Read the model definition and answer for the solid it produces. Units are mm, in the model's axes. Face numbers are marked on the shaded views. Coordinates: 2 decimals unless noted, no trailing zeros. Write each loop counter-clockwise with the first axis right and the second up, starting at its lowest first coordinate (ties: lowest second). Pieces come first, ordered by that corner, then holes.
(1) Section B-B on y = 0 is taken. Write down the section's boundary in (x, z).
(2) Section D-D on z = -10.5 is taken. Write down the section's boundary in (x, y).
(3) Section A-A on x = 10 is taken. Write down the section's boundary in (y, z), then the cut area to 3 significant figures.
(4) Find the intervals of material crossed by probe 1 along Z at (x, y) = (10, 0); probe 2 along X at (y, z) = (0.75, -9); probe 3 along Z at (x, y) = (10, 1), in increasing order.
(5) Section C-C on x = 12 is taken. Write down the section's boundary in (y, z).
(6) The mould has two halves that part along Z. Classify the marked faces 1, 2, 3 and 4: +Z half, -Z half, draft (parallel to the pull), parting line (faces both ways), or undercut.
(7) Given pin 1 (1.6 mm diameter, centred on x = 11.5, z = -13.5, fed in from +Y); pin 2 (0.5 mm diameter, centred on x = 8.5, y = 0, fed in from -Z); pin 3 (1.2 mm diameter, centred on x = 9, z = -13, fed in from -Y), each flat-ended and moving along its own axis, determine where each tip first touches the part or whether it passes through.
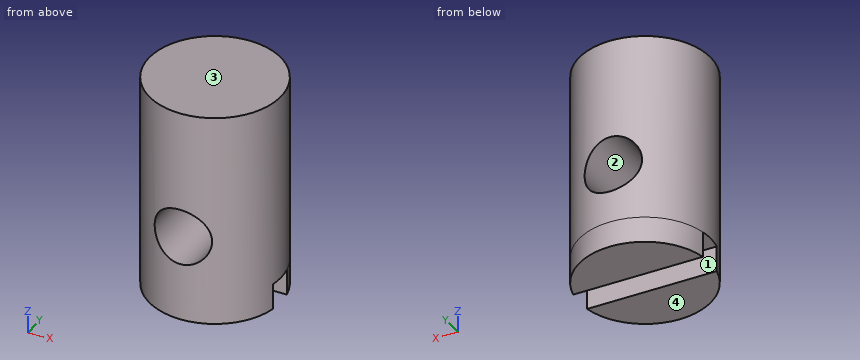
from build123d import *
from build123d.topology import SkipClean

# Parameters (mm, degrees)
SCHIZZO1_W                   = 3.8
SCHIZZO1_H                   = 12.5
TAGLIO_ESTRUSIONE1_START     = -1.5
TAGLIO_ESTRUSIONE1_DEPTH     = 1.5
ESTRUSIONE_ESTRUSIONE1_DEPTH = 1.5
FORO_3_3_3_3_1_D             = 3.3


with BuildPart() as part:
    # Schizzo1 → Rivoluzione1 (revolve)
    with BuildSketch(Plane.XZ, mode=Mode.PRIVATE) as rivoluzione1_sk:
        with Locations((11.9, -7.75)):
            Rectangle(SCHIZZO1_W, SCHIZZO1_H)
    revolve(rivoluzione1_sk.sketch.rotate(Axis((10, 0, -1.5), (0, 0, -1)), 180), axis=Axis((10, 0, -1.5), (0, 0, -1)))

    # Schizzo2 → Taglio-Estrusione1 (cut)
    with BuildSketch(Plane(origin=(0, 0, -14), x_dir=(-1, 0, 0), z_dir=(0, 0, -1)).offset(TAGLIO_ESTRUSIONE1_START)):
        with BuildLine():
            Line((-13.725251669, -0.75), (-6.274748331, -0.75))
            ThreePointArc((-6.274748331, -0.75), (-10, 3.8), (-13.725251669, -0.75))
        make_face()
    extrude(amount=TAGLIO_ESTRUSIONE1_DEPTH, mode=Mode.SUBTRACT)

    # Schizzo3 → Estrusione-Estrusione1 (add)
    with SkipClean():  # the faces are left unmerged after this step: merging them gives an invalid solid
        with BuildSketch(Plane(origin=(0, 0, -12.5), x_dir=(-1, 0, 0), z_dir=(0, 0, -1))):
            with BuildLine():
                Line((-6.274748331, 0.75), (-13.725251669, 0.75))
                ThreePointArc((-13.725251669, 0.75), (-10, 3.8), (-6.274748331, 0.75))
            make_face()
        extrude(amount=ESTRUSIONE_ESTRUSIONE1_DEPTH)

    # Foro Ø3.3 (3.3)-1 (through all)
    with Locations(Plane(origin=(10, 3.8, -9), x_dir=(0, 0, 1), z_dir=(0, 1, 0))):
        with Locations((0, 0)):
            Hole(FORO_3_3_3_3_1_D / 2)


solid = part.part
Response:
1. outline: (6.2, -12.5) - (13.8, -12.5) - (13.8, -1.5) - (6.2, -1.5) - close; hole circle Ø3.3 at (10, -9)
2. outline: (9.31, -3.74) - (9.31, 3.74) arc R3.8 ccw to start; (10.69, -3.74) arc R3.8 ccw to (10.69, 3.74) - close
3. outline: (-3.8, -14) - (-0.75, -14) - (-0.75, -12.5) - (0.75, -12.5) - (0.75, -14) - (3.8, -14) - (3.8, -10.65) - (-3.8, -10.65) - close; (-3.8, -7.35) - (3.8, -7.35) - (3.8, -1.5) - (-3.8, -1.5) - close
3. area: 67.7 mm2
4. probe 1: z = -12.5 to -10.65, -7.35 to -1.5
4. probe 2: x = 6.27 to 8.35, 11.65 to 13.73
4. probe 3: z = -14 to -10.65, -7.35 to -1.5
5. outline: (-3.23, -14) - (-0.75, -14) - (-0.75, -12.5) - (0.75, -12.5) - (0.75, -14) - (3.23, -14) - (3.23, -1.5) - (-3.23, -1.5) - close
6. face 1: draft
6. face 2: undercut
6. face 3: +Z half
6. face 4: -Z half
7. pin 1: stops at y = 3.73
7. pin 2: stops at z = -12.5
7. pin 3: stops at y = -3.78
